For this review, take the finished solid that the model builds, in its own axes (mm). Coordinates: 2 decimals unless noted, no trailing zeros. Write each loop counter-clockwise with the first axis right and the second up, starting at its lowest first coordinate (ties: lowest second). Pieces come first, ordered by that corner, then holes. Notation, with made-up numbers: (87.5, 39.25) - (123.5, 39.25) arc R21 cw to (123.5, 61.25) - close; hole circle Ø7 at (-15, 36). An arc over 180 degrees is marked (long way). Use one line per item in the form item = value. Start each with the question number.
1) Insertion check: P1, Ø1.5, axis at y = 7, z = -1.5, coming from the +X side. The pin has a flat end and moves straight along its axis. Give the tip position at first contact, or say it passes through.
2) We need section D-D (y = 3). Give the boundary of the cut face in (x, z), plus the area to 3 significant figures.
3) For L1, parallel to X at y = 3.25, z = -4.6; L2, parallel to X at y = 5, z = -2.9; L3, parallel to Y at x = 3.5, z = -3.3, list the stretches that pass through material, from the lowest coordinate up. Write a range as from..to.
4) We need section C-C (z = -3.2). Give the boundary of the cut face in (x, y).
5) Mouldability with a two-part tool opening along X and no side actions: class faces 1 (the cylindrical face through (2.02, 3.39, -2.54)), 2 (the flat face through (0, 4, -2)), 3 (the flat face through (12, 4, -5)) as pulls with the +X half, pulls with the -X half, needs draft (parallel to the pull), parting line crosses it, or undercut.
6) We need section A-A (y = 4). Give the boundary of the cut face in (x, z), plus the area to 3 significant figures.
7) We need section B-B (x = 8). Give the boundary of the cut face in (y, z).
```python
from build123d import *

# Parameters (mm, degrees)
SKETCH1_W           = 25
SKETCH1_H           = 5
SKETCH1_R           = 1.6
BOSS_EXTRUDE1_DEPTH = 8
SKETCH2_R           = 1.6
CUT_EXTRUDE1_DEPTH  = 8
FILLET1_R           = 2


with BuildPart() as part:
    # Sketch1 → Boss-Extrude1 (new body)
    with BuildSketch(Plane(origin=(0, 0, 0), x_dir=(1, 0, 0), z_dir=(0, 1, 0))):
        with Locations((12.5, 2.5)):
            Rectangle(SKETCH1_W, SKETCH1_H)
        with Locations(Location((8, 2.5, 0), (0, 0, 270))):
            Circle(SKETCH1_R, mode=Mode.SUBTRACT)
        with Locations(Location((17, 2.5, 0), (0, 0, 270))):
            Circle(SKETCH1_R, mode=Mode.SUBTRACT)
    extrude(amount=BOSS_EXTRUDE1_DEPTH)

    # Sketch2 → Cut-Extrude1 (cut)
    with BuildSketch(Plane(origin=(0, 0, -5), x_dir=(-1, 0, 0), z_dir=(0, 0, -1))):
        with Locations((-21.5, 4)):
            Circle(SKETCH2_R)
        with Locations((-3.5, 4)):
            Circle(SKETCH2_R)
    extrude(amount=-CUT_EXTRUDE1_DEPTH, mode=Mode.SUBTRACT)

    # Fillet1
    fillet1_edges = [part.edges().sort_by_distance(p)[0] for p in [
        (25, 8, -2.5),
        (0, 8, -2.5),
        (25, 0, -2.5),
        (0, 0, -2.5),
    ]]
    fillet(fillet1_edges, radius=FILLET1_R)


solid = part.part
```
Determined:
q1.P1 = 24.98
q2.outline = (0, -5) - (2.25, -5) - (2.25, 0) - (0, 0) - close; (4.75, -5) - (20.25, -5) - (20.25, 0) - (4.75, 0) - close; (22.75, -5) - (25, -5) - (25, 0) - (22.75, 0) - close; hole circle Ø3.2 at (8, -2.5); hole circle Ø3.2 at (17, -2.5)
q2.area = 83.9 mm²
q3.L1 = 0..2.09, 4.91..20.09, 22.91..25
q3.L2 = 0..2.25, 4.75..6.45, 9.55..15.45, 18.55..20.25, 22.75..25
q3.L3 = 0..2.4, 5.6..8
q4.outline = (0, 2) arc R2 ccw to (2, 0) - (6.56, 0) - (6.56, 8) - (2, 8) arc R2 ccw to (0, 6) - close; (9.44, 0) - (15.56, 0) - (15.56, 8) - (9.44, 8) - close; (18.44, 0) - (23, 0) arc R2 ccw to (25, 2) - (25, 6) arc R2 ccw to (23, 8) - (18.44, 8) - close; hole circle Ø3.2 at (3.5, 4); hole circle Ø3.2 at (21.5, 4)
q5.face_1 = undercut
q5.face_2 = pulls with the -X half
q5.face_3 = needs draft
q6.outline = (0, -5) - (1.9, -5) - (1.9, 0) - (0, 0) - close; (5.1, -5) - (19.9, -5) - (19.9, 0) - (5.1, 0) - close; (23.1, -5) - (25, -5) - (25, 0) - (23.1, 0) - close; hole circle Ø3.2 at (8, -2.5); hole circle Ø3.2 at (17, -2.5)
q6.area = 76.9 mm²
q7.outline = (0, -5) - (8, -5) - (8, -4.1) - (0, -4.1) - close; (0, -0.9) - (8, -0.9) - (8, 0) - (0, 0) - close
